The model under review builds one solid part; all positions refer to its coordinate system, in mm. Round coordinates to 2 decimals unless told otherwise and drop trailing zeros. Write each loop counter-clockwise with the first axis right and the second up, starting at its lowest first coordinate (ties: lowest second). Pieces come first, ordered by that corner, then holes. Notation, with made-up numbers: (45, 87.25) -> (54, 87.25) arc R21 ccw to (54, 123.25) -> close; hole circle Ø11 at (-13.5, 89.5). An arc over 180 degrees is marked (long way). Answer as a JSON object with one key per item and string values. Group by question number.
1) To check wall thickness, follow probe 1 along Z at (x, y) = (3.5, 0.5); probe 2 along Y at (x, z) = (-3, -34); probe 3 along X at (y, z) = (-0.25, 3). State the ranges of each line that lie inside material, in increasing order. Write a range as [from, to].
2) Insertion check: pin 1 Ø4 at (x, z) = (3, -2) entering from +Y; pin 2 Ø1.5 at (x, z) = (-2.5, 54.5) entering from +Y. Each pin has a flat end and moves straight along its axis. Give the tip position at first contact, or say it passes through.
3) We need section B-B, the plane z = 57. Write out the cut boundary in (x, y).
4) We need section A-A, the plane z = 123. Write out the cut boundary in (x, y).
from build123d import *

# Parameters (mm, degrees)
SKETCH_1_R          = 5
EXTRUDE_1_DEPTH     = 60
SKETCH_2_R          = 3.5
EXTRUDE_2_DEPTH     = 2
EXTRUDE_START       = 2
SKETCH_3_R          = 3.5
EXTRUDE_3_DEPTH     = 2
EXTRUDE_START_2     = 90
SKETCH_4_R          = 5
EXTRUDE_4_DEPTH     = 90
SKETCH_5_R          = 5
EXTRUDE_5_DEPTH     = 90
CUT_EXTRUDE_START   = -40
SKETCH_6_R          = 5
SKETCH_6_R_2        = 4
CUT_EXTRUDE_2_DEPTH = 40
SKETCH_7_R          = 5
SKETCH_7_R_2        = 4
CUT_EXTRUDE_3_DEPTH = 40
CUT_EXTRUDE_START_2 = 2
SKETCH_8_R          = 5
SKETCH_8_R_2        = 3.5
CUT_EXTRUDE_4_DEPTH = 2
SKETCH_9_R          = 5
SKETCH_9_R_2        = 3.5
CUT_EXTRUDE_5_DEPTH = 2


with BuildPart() as part:
    # 草图1 → 凸台-拉伸1 (new body)
    with BuildSketch(Plane.XY):
        Circle(SKETCH_1_R)
    extrude(amount=EXTRUDE_1_DEPTH)

    # 草图2 → 凸台-拉伸2 (add)
    with BuildSketch(Plane.XY.offset(60)):
        Circle(SKETCH_2_R)
    extrude(amount=EXTRUDE_2_DEPTH)

    # 草图3 → 凸台-拉伸3 (add)
    with BuildSketch(Plane(origin=(0, 0, 0), x_dir=(-1, 0, 0), z_dir=(0, 0, -1)).offset(EXTRUDE_START)):
        with Locations(Location((0, 0, 0), (0, 0, 180))):
            Circle(SKETCH_3_R)
    extrude(amount=-EXTRUDE_3_DEPTH)

    # 草图4 → 凸台-拉伸4 (add)
    with BuildSketch(Plane(origin=(0, 0, -2), x_dir=(-1, 0, 0), z_dir=(0, 0, -1)).offset(EXTRUDE_START_2)):
        with Locations(Location((0, 0, 0), (0, 0, 180))):
            Circle(SKETCH_4_R)
    extrude(amount=-EXTRUDE_4_DEPTH)

    # 草图5 → 凸台-拉伸5 (add)
    with BuildSketch(Plane.XY.offset(62)):
        Circle(SKETCH_5_R)
    extrude(amount=EXTRUDE_5_DEPTH)

    # 草图6 → 切除-拉伸2 (cut)
    with BuildSketch(Plane.XY.offset(152).offset(CUT_EXTRUDE_START)):
        with Locations(Location((0, 0, 0), (0, 0, 180))):
            Circle(SKETCH_6_R)
        Circle(SKETCH_6_R_2, mode=Mode.SUBTRACT)
    extrude(amount=CUT_EXTRUDE_2_DEPTH, mode=Mode.SUBTRACT)

    # 草图7 → 切除-拉伸3 (cut)
    with BuildSketch(Plane(origin=(0, 0, -92), x_dir=(-1, 0, 0), z_dir=(0, 0, -1))):
        with Locations(Location((0, 0, 0), (0, 0, 180))):
            Circle(SKETCH_7_R)
        with Locations(Location((0, 0, 0), (0, 0, 180))):
            Circle(SKETCH_7_R_2, mode=Mode.SUBTRACT)
    extrude(amount=-CUT_EXTRUDE_3_DEPTH, mode=Mode.SUBTRACT)

    # 草图8 → 切除-拉伸4 (cut)
    with BuildSketch(Plane(origin=(0, 0, -42.5), x_dir=(-1, 0, 0), z_dir=(0, 0, -1)).offset(CUT_EXTRUDE_START_2)):
        with Locations(Location((0, 0, 0), (0, 0, 180))):
            Circle(SKETCH_8_R)
        with Locations(Location((0, 0, 0), (0, 0, 180))):
            Circle(SKETCH_8_R_2, mode=Mode.SUBTRACT)
    extrude(amount=-CUT_EXTRUDE_4_DEPTH, mode=Mode.SUBTRACT)

    # 草图9 → 切除-拉伸5 (cut)
    with BuildSketch(Plane.XY.offset(102.5)):
        with Locations(Location((0, 0, 0), (0, 0, 180))):
            Circle(SKETCH_9_R)
        Circle(SKETCH_9_R_2, mode=Mode.SUBTRACT)
    extrude(amount=CUT_EXTRUDE_5_DEPTH, mode=Mode.SUBTRACT)


solid = part.part
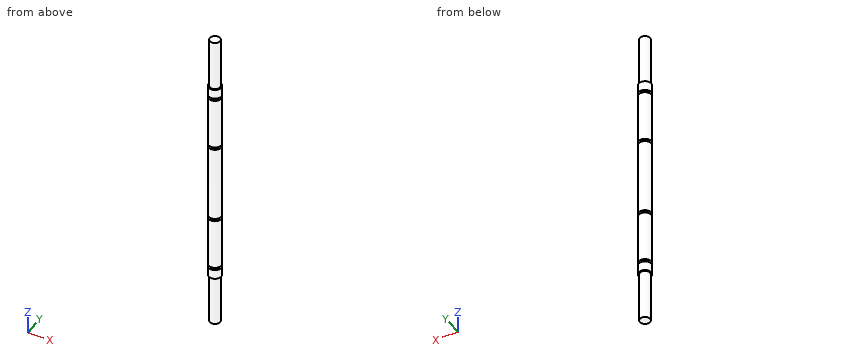
Here are the results:
{
 "1": {"probe 1": "z = [-92, -44.5], [-42.5, -2], [0, 60], [62, 102.5], [104.5, 152]", "probe 2": "y = [-4, 4]", "probe 3": "x = [-4.99, 4.99]"},
 "2": {"pin 1": "stops at y = 4.9", "pin 2": "stops at y = 4.68"},
 "3": {"outline": "circle Ø10 at (0, 0)"},
 "4": {"outline": "circle Ø8 at (0, 0)"}
}
